from build123d import *

# Parameters (mm, degrees)
F0_W     = 70
F0_H     = 83
F1_DEPTH = 4
F2_R     = 12.5
F2_R_2   = 11
F3_DEPTH = 44
F5_DEPTH = 11.25
F6_R     = 4
F7_DEPTH = 25


with BuildPart() as f1:
    # F0 (on Top) → F1 (new body)
    with BuildSketch(Plane.XY):
        Rectangle(F0_W, F0_H)
    extrude(amount=-F1_DEPTH)

    # F2 (on face) → F3 (join)
    with BuildSketch(Plane.XY):
        Circle(F2_R)
        Circle(F2_R_2, mode=Mode.SUBTRACT)
    extrude(amount=F3_DEPTH)

    # F4 (on Front) → F5 (cut, symmetric)
    with BuildSketch(Plane.XZ):
        with BuildLine():
            Line((10.5089721754, 44), (-10.4910278246, 44))
            ThreePointArc((-10.4910278246, 44), (0.0089721754, 41.7379000772), (10.5089721754, 44))
        make_face()
        with BuildLine():
            Line((-10.4910278246, 44), (-12.4910278246, 44))
            ThreePointArc((-12.4910278246, 44), (0.0089721754, 40.9948974278), (12.5089721754, 44))
            Line((12.5089721754, 44), (10.5089721754, 44))
            ThreePointArc((10.5089721754, 44), (0.0089721754, 41.7379000772), (-10.4910278246, 44))
        make_face()
    extrude(amount=F5_DEPTH, both=True, mode=Mode.SUBTRACT)

    # F6 (on face) → F7 (cut)
    with BuildSketch(Plane(origin=(0, 0, -4), x_dir=(1, 0, 0), z_dir=(0, 0, -1))):
        with Locations((-15, 27.5)):
            Circle(F6_R)
        with Locations((15, 27.5)):
            Circle(F6_R)
        with Locations((15, -25.5)):
            Circle(F6_R)
        with Locations((-15, -25.5)):
            Circle(F6_R)
    extrude(amount=-F7_DEPTH, mode=Mode.SUBTRACT)

    # F9: sweep along a path in F8
    with BuildLine(Plane.YZ) as f9_path:
        Line((50, 37), (-50, 37))
    # F4 (on Front) → F9 (sweep)
    with BuildSketch(Plane.XZ):
        with BuildLine():
            Line((-10.4910278246, 44), (-12.4910278246, 44))
            ThreePointArc((-12.4910278246, 44), (0.0089721754, 40.9948974278), (12.5089721754, 44))
            Line((12.5089721754, 44), (10.5089721754, 44))
            ThreePointArc((10.5089721754, 44), (0.0089721754, 41.7379000772), (-10.4910278246, 44))
        make_face()
    sweep(path=f9_path.line)


solid = f1.part
Check sheet for the modelled part. Datum: model origin and axes. Units: mm. A direction names the side the tool comes from. Round coordinates to 2 decimals unless told otherwise and drop trailing zeros. Order: outer loops, then holes, each group sorted by start corner. A loop starts at its lowest first (then second) coordinate and runs counter-clockwise, first axis right, second up.
Q1. Cross-section at D-D, the plane y = 25.5. Enter the section's corners in (x, z), plus the area to 3 significant figures.
Filled sheet:
outline: (-35, -4) - (-19, -4) - (-19, 0) - (-35, 0) - close; (-12.49, 44) arc R27.5 ccw to (12.51, 44) - (10.51, 44) arc R25.5 cw to (-10.49, 44) - close; (-11, -4) - (11, -4) - (11, 0) - (-11, 0) - close; (19, -4) - (35, -4) - (35, 0) - (19, 0) - close
area: 235 mm2
Q2. Draft check along X on faces 1 (the face through (-35, -1, -2)), 2 (the face through (0.1, -50, 41.5)), 3 (the face through (0, 11.25, 43)), 4 (the face through (-5.894, -11.811, 41.636)). Enter one of: pulls with the +X half, pulls with the -X half, needs draft (parallel to the pull), parting line crosses it, or undercut.
Filled sheet:
face 1: pulls with the -X half
face 2: needs draft
face 3: undercut
face 4: parting line crosses it
Q3. Cross-section at B-B, the plane x = 0. Enter the section's corners in (y, z), plus the area to 3 significant figures.
Filled sheet:
outline: (-50, 40.99) - (-12.5, 40.99) - (-12.5, 0) - (-41.5, 0) - (-41.5, -4) - (41.5, -4) - (41.5, 0) - (12.5, 0) - (12.5, 40.99) - (50, 40.99) - (50, 41.74) - (12.5, 41.74) - (12.5, 44) - (11.25, 44) - (11.25, 41.74) - (-11.25, 41.74) - (-11.25, 44) - (-12.5, 44) - (-12.5, 41.74) - (-50, 41.74) - close; hole (-11, 0) - (11, 0) - (11, 40.99) - (-11, 40.99) - close
area: 535 mm2
Q4. Depth check by flat-ended pin: P1, Ø2, axis at x = 5, z = -1.5, coming from the +Y side; P2, Ø12, axis at x = -6, y = 8.5, coming from the +Z side; P3, Ø2, axis at x = 10.5, z = -2, coming from the -Y side; P4, Ø12, axis at x = 13.5, z = 19.5, coming from the +Y side. Enter the tip coordinate at first touch or a pass-through.
Filled sheet:
P1: stops at y = 41.5
P2: stops at z = 44
P3: stops at y = -41.5
P4: stops at y = 10
Q5. Set-up check for faces 5 (the face through (12.05, 22.8, -2.03)), 6 (the face through (-2.38, -10.74, 21.34)), 7 (the face through (-0.1, -12.5, 42.9)), 8 (the face through (0, -41.5, -2)), 9 (the face through (0, -11.25, 43)): record each of +Z, -Z, +X, -X, +Y, -Y from which the full face is reachable in a straight line by a thin tool's end or side.
Filled sheet:
face 5: -Z
face 6: none
face 7: +Z, -Y
face 8: -Z, +X, -X, -Y
face 9: +Z
Q6. Scan lines: L1, parallel to X at y = 25.5, z = -0.95; L2, parallel to Y at x = 15, z = -1; L3, parallel to Z at x = 0.5, y = 14.5. Record each from-to range of solid material in increasing order.
Filled sheet:
L1: x = -35 to -19, -11 to 11, 19 to 35
L2: y = -41.5 to -31.5, -23.5 to 21.5, 29.5 to 41.5
L3: z = -4 to 0, 41 to 41.74
Q7. Cross-section at C-C, the plane x = -15. Enter the section's corners in (y, z).
Filled sheet:
outline: (-41.5, -4) - (-31.5, -4) - (-31.5, 0) - (-41.5, 0) - close; (-23.5, -4) - (21.5, -4) - (21.5, 0) - (-23.5, 0) - close; (29.5, -4) - (41.5, -4) - (41.5, 0) - (29.5, 0) - close
Q8. Cross-section at A-A, the plane y = -33. Enter the section's corners in (x, z), plus the area to 3 significant figures.
Filled sheet:
outline: (-35, -4) - (35, -4) - (35, 0) - (-35, 0) - close; (-12.49, 44) arc R27.5 ccw to (12.51, 44) - (10.51, 44) arc R25.5 cw to (-10.49, 44) - close
area: 299 mm2
